Read the model definition and answer for the solid it produces. Units are mm, in the model's axes. Face numbers are marked on the shaded views. A direction names the side the tool comes from. Coordinates: 2 decimals unless noted, no trailing zeros. Write each loop counter-clockwise with the first axis right and the second up, starting at its lowest first coordinate (ties: lowest second). Pieces come first, ordered by that corner, then holes. Notation, with made-up numbers: M 25.25,70 L 34.25,70 A28 cw 34.25,106 Z; hole C 85.5,46.25 d2. An arc over 180 degrees is marked long. Write item = value, one per line.
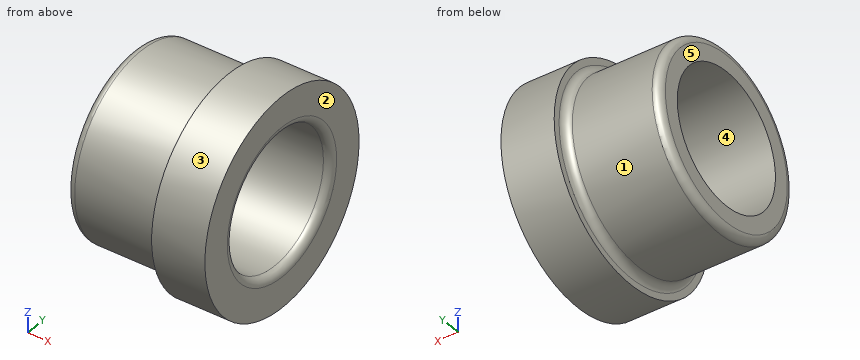
from build123d import *

# Parameters (mm, degrees)
F2_R = 2
F3_R = 2


with BuildPart() as f1:
    # F0 (on Top) → F1 (revolve)
    with BuildSketch(Plane.XY):
        Polygon((0, 17.5), (0, 27.5), (-14, 27.5), (-14, 23.75), (-39, 23.75), (-39, 17.5), align=None)
    revolve(axis=Axis((-10.876282, 0, 0), (1, 0, 0)))

    # F2
    f2_edges = [f1.edges().sort_by_distance(p)[0] for p in [
        (-14, -23.75, 0),
    ]]
    fillet(f2_edges, radius=F2_R)

    # F3
    f3_edges = [f1.edges().sort_by_distance(p)[0] for p in [
        (-39, -23.75, 0),
        (0, -17.5, 0),
    ]]
    fillet(f3_edges, radius=F3_R)


solid = f1.part
Item 1: For a pull along Y with two mould halves and no side action, classify the marked faces 3, 4 and 5 as released by +Y, released by -Y, zero draft, split by the parting line, or undercut.
Worked answers:
face_3 = split by the parting line
face_4 = undercut
face_5 = zero draft
Item 2: Flat-ended cylindrical pins translate along their axes: pin 1 (12 mm diameter, centred on x = -27, y = 6, fed in from -Z); pin 2 (1 mm diameter, centred on x = -34, y = 18.5, fed in from -Z); pin 3 (5 mm diameter, centred on x = -29.5, z = -13.5, fed in from +Y). Find the tip coordinate at first contact, or state that the pin passes through.
Worked answers:
pin_1 = -23.75
pin_2 = -15.49
pin_3 = 21.05
Item 3: Find section D-D (x = -19). Determine the outline of the cut face in (y, z), and give its area (3 significant figures).
Worked answers:
outline = C 0,0 d47.5; hole C 0,0 d35
area = 810 mm²
Item 4: Consider line 1 along Z through (x, y) = (-19.5, 0); line 2 along Y through (x, z) = (-10, 14); line 3 along Y through (x, z) = (-26.5, 16). Determine where each line is inside the solid, lowest interval first. Write a range as from..to.
Worked answers:
line_1 = -23.75..-17.5, 17.5..23.75
line_2 = -23.67..-10.5, 10.5..23.67
line_3 = -17.55..-7.09, 7.09..17.55
Item 5: Find section A-A (y = 0). Determine the outline of the cut face in (x, z).
Worked answers:
outline = M -39,-21.75 A2 ccw -37,-23.75 L -16,-23.75 A2 cw -14,-25.75 L -14,-27.5 L 0,-27.5 L 0,-19.5 A2 ccw -2,-17.5 L -39,-17.5 Z; M -39,17.5 L -2,17.5 A2 ccw 0,19.5 L 0,27.5 L -14,27.5 L -14,25.75 A2 cw -16,23.75 L -37,23.75 A2 ccw -39,21.75 Z
Item 6: Which of the six approach directions +Z, -Z, +X, -X, +Y, -Y give full straight-line access (tool end or side, diameter ignored) to the marked faces 1 and 2?
Worked answers:
face_1 = -X
face_2 = +Z, -Z, +X, +Y, -Y
Item 7: Find section C-C (x = -5.5). Determine the outline of the cut face in (y, z).
Worked answers:
outline = C 0,0 d55; hole C 0,0 d35
